Answer from the drawing. Dimensions are ordinates in mm from the lowest x, y and z of the part. Coordinates: 2 decimals unless noted, no trailing zeros. Write each loop counter-clockwise with the first axis right and the second up, starting at its lowest first coordinate (ties: lowest second). Pieces come first, ordered by that corner, then holes. Notation, with made-up numbers: (-23, 49) -> (-5, 49) arc R18 cw to (-5, 53) -> close; hole circle Ø10 at (60.5, 52). An arc over 180 degrees is marked (long way). Use CSV: the item, a comma, the result in double quotes.
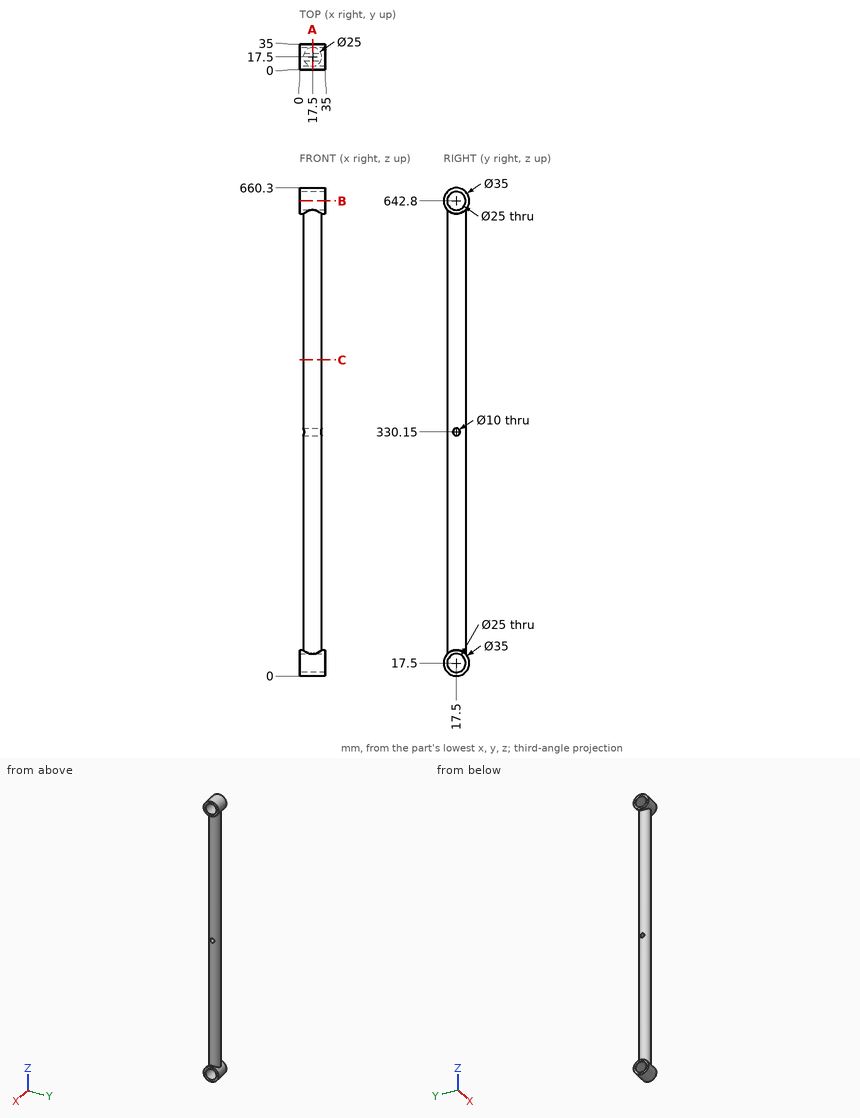
1. Find the intervals of material crossed by line 1 along Z through (x, y) = (25, 17); line 2 along Y through (x, z) = (14.5, 642.8); line 3 along Z through (x, y) = (20, 9), in increasing order.
Solutions:
line 1,"z = 0.01 to 5.01, 29.99 to 325.18, 335.12 to 630.31, 655.29 to 660.29"
line 2,"y = 0 to 5, 30 to 35"
line 3,"z = 2.2 to 8.33, 26.67 to 633.63, 651.97 to 658.1"
2. A cutting plane is placed at C-C (z = 427.5). Give the vertices of the cut face in (x, y), and give its area (3 significant figures).
Solutions:
outline,"circle Ø25 at (17.5, 17.5)"
area,"491 mm^2"
3. A cutting plane is placed at A-A (x = 17.5). Give the vertices of the cut face in (y, z), and give its area (3 significant figures).
Solutions:
outline,"(5, 29.75) arc R17.5 ccw (long way) to (30, 29.75) -> (30, 630.55) arc R17.5 ccw (long way) to (5, 630.55) -> close; hole circle Ø25 at (17.5, 17.5); hole circle Ø25 at (17.5, 642.8); hole circle Ø10 at (17.5, 330.15)"
area,"15,700 mm^2"
4. A cutting plane is placed at B-B (z = 642.8). Give the vertices of the cut face in (x, y), and give its area (3 significant figures).
Solutions:
outline,"(0, 0) -> (35, 0) -> (35, 5) -> (0, 5) -> close; (0, 30) -> (35, 30) -> (35, 35) -> (0, 35) -> close"
area,"350 mm^2"
5. Each of these flat-tipped pins is pushed along its axis until it touches: pin 1 Ø1.5 at (y, z) = (28, 477) entering from +X; pin 2 Ø12 at (x, z) = (10, 349) entering from -Y; pin 3 Ø6 at (x, z) = (16.5, 267.5) entering from +Y. Where does it stop, or does it pass through?
Solutions:
pin 1,"stops at x = 25.32"
pin 2,"stops at y = 5.09"
pin 3,"stops at y = 30"
